Autodesk Inventor part; units mm, degrees
ref_plane "Work Plane2" through (-350.7586, -218.6666, 34.497) normal (0, 0, -1) x (-0.0253, 0.9997, 0)
ref_plane "YZ Plane" through (0, 0, 0) normal (1, 0, 0) x (0, 1, 0)
ref_plane "XZ Plane" through (0, 0, 0) normal (0, 1, 0) x (-1, 0, 0)
ref_plane "Work Plane1" through (0, 0, 0) normal (0, 0, 1) x (1, 0, 0)
sketch "Sketch1" plane through (0, 0, 0) normal (0, 0, 1) x (1, 0, 0)
  circle A0 centre (0.445, -8.7) radius 2.25 construction
  circle A1 centre (0.445, -8.7) radius 2.25
  line L0 (3.62, -5.525) -> (-2.73, -5.525)
  line L1 (-2.73, -5.525) -> (-2.73, -11.875)
  line L2 (3.62, -5.525) -> (-2.73, -11.875) construction
  arc A2 (1.27, -12.7) -> (4.445, -9.525) centre (1.27, -9.525) ccw construction
  arc A3 (2.9413, -11.875) -> (3.62, -11.1963) centre (0.445, -8.7) ccw
  line L3 (3.62, -11.1963) -> (3.62, -5.525)
  line L4 (-2.73, -11.875) -> (2.9413, -11.875)
  point P0 (0, 0)
  dimension "d1" = 6.35
ref_plane "Work Plane2" through (-350.7586, -218.6666, 34.497) normal (0, 0, -1) x (-0.0253, 0.9997, 0)
extrude "Extrusion1" add sketch "Sketch1" along normal up to surface (34.497 mm away)
properties part number "odometry standoff"
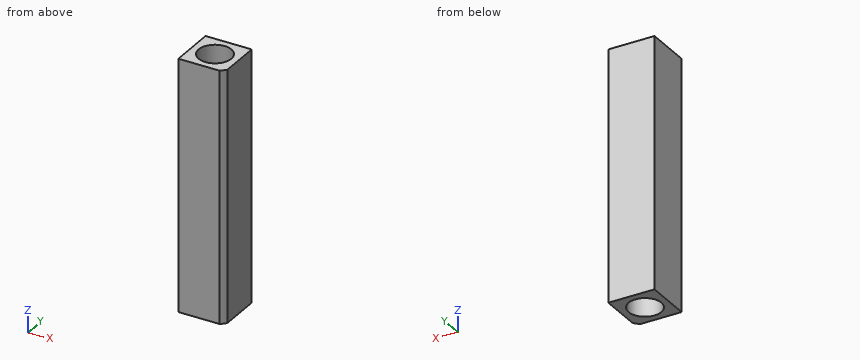
For this review, take the finished solid that the model builds, in its own axes (mm). Round coordinates to 2 decimals unless told otherwise and drop trailing zeros. Write each loop counter-clockwise with the first axis right and the second up, starting at its lowest first coordinate (ties: lowest second). Pieces come first, ordered by that corner, then holes. Notation, with made-up numbers: (-37, -32.75) - (-31, -32.75) arc R15 cw to (-31, -23.75) - close; hole circle Ø2 at (64.25, -21.5). An arc over 180 degrees is marked (long way). Answer as CSV lines item,"result". Start each with the question number.
(1) Add section C-C, the plane x = -0.5. State the section outline as (y, z) points (3 decimals).
(2) For line 1 (Y direction, x = 0.5, z = 11.5) (3 decimals); line 2 (X direction, y = -7.75, z = 11); line 3 (Y direction, x = -0.75, z = 17.5) (3 decimals), list the stretches that pass through material, from the lowest coordinate up.
(3) Add section B-B, the plane z = 9. State the section outline as (x, y) points (3 decimals), plus the area to 3 significant figures.
(4) Add section A-A, the plane y = -8.7. State the section outline as (x, z) points (3 decimals), plus the area to 3 significant figures.
From the geometry:
1,outline,"(-11.875, 0) - (-10.742, 0) - (-10.742, 34.497) - (-11.875, 34.497) - close; (-6.658, 0) - (-5.525, 0) - (-5.525, 34.497) - (-6.658, 34.497) - close"
2,line 1,"y = -11.875 to -10.949, -6.451 to -5.525"
2,line 2,"x = -2.73 to -1.59, 2.48 to 3.62"
2,line 3,"y = -11.875 to -10.606, -6.794 to -5.525"
3,outline,"(-2.73, -11.875) - (2.941, -11.875) arc R4.039 ccw to (3.62, -11.196) - (3.62, -5.525) - (-2.73, -5.525) - close; hole circle Ø4.5 at (0.445, -8.7)"
3,area,"24.2 mm²"
4,outline,"(-2.73, 0) - (-1.805, 0) - (-1.805, 34.497) - (-2.73, 34.497) - close; (2.695, 0) - (3.62, 0) - (3.62, 34.497) - (2.695, 34.497) - close"
4,area,"63.8 mm²"
